Geometry: final body of the model. Coordinates: model frame, mm. Face numbers are marked on the shaded views. Coordinates: 2 decimals unless noted, no trailing zeros. Loops run counter-clockwise (first coordinate to the right, second up) from the corner with the lowest first, then second, coordinate; pieces in that order, holes last. Notation, with made-up numbers: (-5.75, 15.5) - (16.25, 15.5) arc R30 cw to (16.25, 46.5) - close; hole circle Ø7 at (-30.5, -25.5). An arc over 180 degrees is marked (long way). Return JSON: item names as keys, results as strings.
Autodesk Inventor part; units mm, degrees
ref_plane "YZ Plane" through (0, 0, 0) normal (1, 0, 0) x (0, 1, 0)
ref_plane "XZ Plane" through (0, 0, 0) normal (0, 1, 0) x (-1, 0, 0)
ref_plane "XY Plane" through (0, 0, 0) normal (0, 0, 1) x (1, 0, 0)
sketch "Sketch9" plane through (0, 0, 0) normal (0, 1, 0) x (-1, 0, 0)
  line L0 (15, 15) -> (-15, 15)
  line L1 (-15, 15) -> (-15, -15)
  line L2 (-15, -15) -> (15, -15)
  line L3 (15, -15) -> (15, 15)
  line L4 (15, 15) -> (-15, -15) construction
  line L5 (-15, 15) -> (15, -15) construction
  line L6 (-13, 13) -> (13, 13)
  line L7 (13, 13) -> (13, -13)
  line L8 (13, -13) -> (-13, -13)
  line L9 (-13, -13) -> (-13, 13)
  point P0 (0, 0)
  dimension "d172" = 30
  dimension "d173" = 30
  dimension "d174" = 2
extrude "Extrusion3" add sketch "Sketch9" against normal blind 430
sketch "Sketch10" plane through (0, 0, 0) normal (1, 0, 0) x (0, 1, 0)
  line L0 (0, 15) -> (0, -15) construction
  line L1 (0, 15) -> (-430, 15) construction
  line L2 (-430, -15) -> (-430, 15) construction
  line L3 (0, -15) -> (-430, -15) construction
  line L4 (-412, 8.5) -> (-395, 8.5)
  line L5 (-395, 8.5) -> (-395, -8.5)
  line L6 (-395, -8.5) -> (-412, -8.5)
  line L7 (-412, -8.5) -> (-412, 8.5)
  line L8 (-412, 8.5) -> (-395, -8.5) construction
  line L9 (-395, 8.5) -> (-412, -8.5) construction
  circle A0 centre (-403.5, 0) radius 8.5
  line L10 (0, 15) -> (0, -15)
  point P0 (0, 0)
  point P1 (0, 0)
  point P2 (-430, 0)
  dimension "d177" = 17
  dimension "d178" = 17
  dimension "d191" = 18
extrude "Extrusion4" cut sketch "Sketch10" along normal through all contours A0
pattern_linear "Rectangular Pattern4" count 4 spacing 120 along (0, 1, 0) of "Extrusion4"
properties part number "ANP 1436 FDS WAY tube6" material "Stainless Steel"
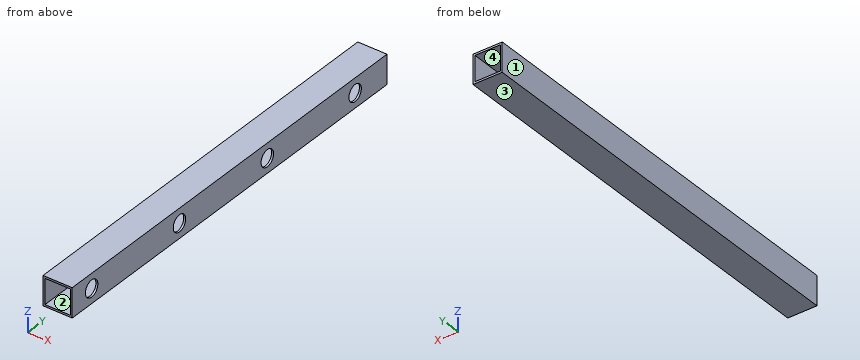
Item 1: Section query C-C, the plane x = -4.75. Return loops of the section in (y, z).
Worked out:
{"outline": "(-430, -15) - (0, -15) - (0, -13) - (-430, -13) - close; (-430, 13) - (0, 13) - (0, 15) - (-430, 15) - close"}
Item 2: First-contact query: pin 1 Ø12 at (x, z) = (-3, -0.5) entering from +Y; pin 2 Ø15.5 at (y, z) = (-403.5, 0) entering from +X. Flat tips, straight axial feed; report the tip coordinate or a pass-through.
Worked out:
{"pin 1": "through", "pin 2": "x = -13"}
Item 3: Ray query, probe 1 along Y at (x, z) = (13.5, 0); probe 2 along X at (y, z) = (-199.5, -4.75). Return the intervals inside material, ascending. Write a range as from..to.
Worked out:
{"probe 1": "-430..-412, -395..-292, -275..-172, -155..-52, -35..0", "probe 2": "-15..-13, 13..15"}
Item 4: Section query A-A, the plane z = 0. Return loops of the section in (x, y).
Worked out:
{"outline": "(-15, -430) - (-13, -430) - (-13, 0) - (-15, 0) - close; (13, -430) - (15, -430) - (15, -412) - (13, -412) - close; (13, -395) - (15, -395) - (15, -292) - (13, -292) - close; (13, -275) - (15, -275) - (15, -172) - (13, -172) - close; (13, -155) - (15, -155) - (15, -52) - (13, -52) - close; (13, -35) - (15, -35) - (15, 0) - (13, 0) - close"}
Item 5: Section query B-B, the plane y = -80. Return loops of the section in (x, z).
Worked out:
{"outline": "(-15, -15) - (15, -15) - (15, 15) - (-15, 15) - close; hole (-13, -13) - (13, -13) - (13, 13) - (-13, 13) - close"}
Item 6: Mould query, pull axis X, two halves, no side actions, for the marked faces 1, 2, 3 and 4. Classes: +X half, -X half, draft (parallel to the pull), parting line (faces both ways), or undercut.
Worked out:
{"face 1": "-X half", "face 2": "undercut", "face 3": "draft", "face 4": "undercut"}
